Could you check a few things on this drawing? It's one solid part, dimensions in mm from its lowest x, y, z. A direction names the side the tool comes from. Give positions to 0.01 mm unless a question says otherwise; leave off trailing zeros. Loops run counter-clockwise (first coordinate to the right, second up) from the corner with the lowest first, then second, coordinate; pieces in that order, holes last. Notation, with made-up numbers: M 27,-8 L 66,-8 A27 ccw 66,23 Z; hole C -10.5,36 d11. An arc over 180 degrees is marked long. Return JSON: item names as keys, results as strings. Group by question number.
1. For pin 1 (1 mm diameter, centred on x = 9.5, y = 1.5, fed in from +Z); pin 2 (4 mm diameter, centred on y = 4.5, z = 2.5, fed in from +X); pin 3 (4 mm diameter, centred on x = 21.5, z = 2.5, fed in from -Y), each with a flat end and sliding along its axis, tell me the tip position at first contact or that it passes through.
2. If we section it at B-B (z = 4): Write out the boundary of the cut face in (x, y), plus the area to 3 significant figures.
3. If we section it at C-C (y = 6.5): Write out the boundary of the cut face in (x, z).
4. For the marked faces 1 and 2, which set-ups out of +Z, -Z, +X, -X, +Y, -Y let a thin tool reach every point of the face, with its end or its side?
5. If we section it at A-A (x = 29): Write out the boundary of the cut face in (y, z), plus the area to 3 significant figures.
6. If we mould it in two halves opening along Z, with no side actions, what happens to the marked faces 3, 4 and 5? For each: +Z half, -Z half, draft (parallel to the pull), parting line (faces both ways), or undercut.
7. Please list where these lines run through material, in increasing order: line 1 (X direction, y = 6.6, z = 4); line 2 (Y direction, x = 15, z = 3.25); line 3 (X direction, y = 2.25, z = 2.5).
8. If we section it at D-D (z = 1): Write out the boundary of the cut face in (x, y), plus the area to 3 significant figures.
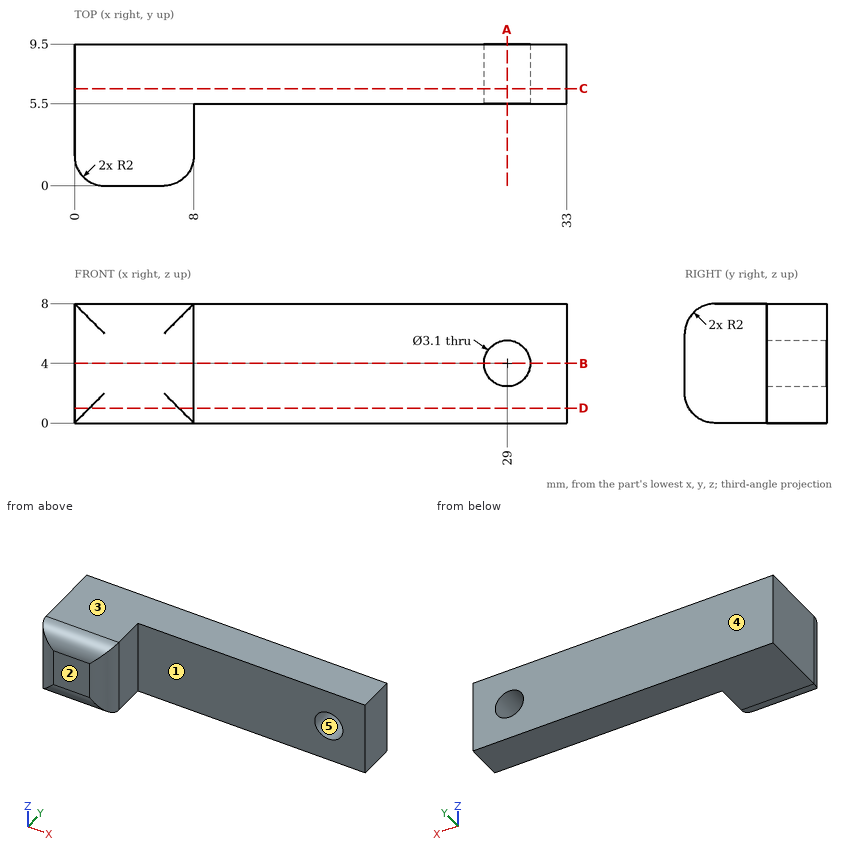
Answer:
{
 "1": {"pin 1": "passes through", "pin 2": "stops at x = 33", "pin 3": "stops at y = 5.5"},
 "2": {"outline": "M 0,2 A2 ccw 2,0 L 6,0 A2 ccw 8,2 L 8,5.5 L 27.45,5.5 L 27.45,9.5 L 0,9.5 Z; M 30.55,5.5 L 33,5.5 L 33,9.5 L 30.55,9.5 Z", "area": "162 mm²"},
 "3": {"outline": "M 0,0 L 33,0 L 33,8 L 0,8 Z; hole C 29,4 d3.1"},
 "4": {"face 1": "+Z, -Z, +X, -Y", "face 2": "+Z, -Z, +X, -X, -Y"},
 "5": {"outline": "M 5.5,0 L 9.5,0 L 9.5,2.45 L 5.5,2.45 Z; M 5.5,5.55 L 9.5,5.55 L 9.5,8 L 5.5,8 Z", "area": "19.6 mm²"},
 "6": {"face 3": "+Z half", "face 4": "draft", "face 5": "undercut"},
 "7": {"line 1": "x = 0 to 27.45, 30.55 to 33", "line 2": "y = 5.5 to 9.5", "line 3": "x = 0 to 8"},
 "8": {"outline": "M 0,2 A2 ccw 1,0.27 L 7,0.27 A2 ccw 8,2 L 8,5.5 L 33,5.5 L 33,9.5 L 0,9.5 Z", "area": "173 mm²"}
}
